```python
from build123d import *

# Parameters (mm, degrees)
SKETCH1_W            = 140
SKETCH1_H            = 92
BOSS_EXTRUDE1_DEPTH  = 6
SKETCH3_R            = 11
SKETCH3_R_2          = 1.6
CUT_EXTRUDE2_DEPTH   = 7
SKETCH6_W            = 10
SKETCH6_H            = 6
CUT_EXTRUDE12_DEPTH  = 4
SKETCH61_W           = 10
SKETCH61_H           = 6
CUT_EXTRUDE14_DEPTH  = 4
SKETCH62_W           = 10
SKETCH62_H           = 6
CUT_EXTRUDE15_DEPTH  = 4
SKETCH63_W           = 10
SKETCH63_H           = 6
CUT_EXTRUDE16_DEPTH  = 4
SKETCH65_W           = 10
SKETCH65_H           = 6
CUT_EXTRUDE17_DEPTH  = 4
SKETCH66_W           = 10
SKETCH66_H           = 6
CUT_EXTRUDE18_DEPTH  = 4
SKETCH67_W           = 10
SKETCH67_H           = 6
CUT_EXTRUDE19_DEPTH  = 4
SKETCH68_W           = 10
SKETCH68_H           = 6
CUT_EXTRUDE110_DEPTH = 4
FILLET1_R            = 5


with BuildPart() as part:
    # Sketch1 → Boss-Extrude1 (new body)
    with BuildSketch(Plane(origin=(0, 0, 0), x_dir=(1, 0, 0), z_dir=(0, 1, 0))):
        Rectangle(SKETCH1_W, SKETCH1_H)
    extrude(amount=BOSS_EXTRUDE1_DEPTH)

    # Sketch3 → Cut-Extrude2 (cut, through all)
    with BuildSketch(Plane(origin=(0, 6, 0), x_dir=(1, 0, 0), z_dir=(0, 1, 0))):
        with Locations((49, 0)):
            Circle(SKETCH3_R)
        with Locations((33.5, -15.5)):
            Circle(SKETCH3_R_2)
        with Locations((33.5, 15.5)):
            Circle(SKETCH3_R_2)
        with Locations((64.5, 15.5)):
            Circle(SKETCH3_R_2)
        with Locations((64.5, -15.5)):
            Circle(SKETCH3_R_2)
    extrude(amount=-CUT_EXTRUDE2_DEPTH, mode=Mode.SUBTRACT)

    # Sketch6 → Cut-Extrude12 (cut, symmetric)
    with BuildSketch(Plane(origin=(49.232221392, 3, -81), x_dir=(1, 0, 0), z_dir=(0, 1, 0))):
        with Locations((0.767778608, -44)):
            Rectangle(SKETCH6_W, SKETCH6_H)
    cut_extrude12 = extrude(amount=CUT_EXTRUDE12_DEPTH, both=True, mode=Mode.SUBTRACT)

    # Sketch61 → Cut-Extrude14 (cut, symmetric)
    with BuildSketch(Plane(origin=(15.898888059, 3, -81), x_dir=(1, 0, 0), z_dir=(0, 1, 0))):
        with Locations((0.767778608, -44)):
            Rectangle(SKETCH61_W, SKETCH61_H)
    cut_extrude14 = extrude(amount=CUT_EXTRUDE14_DEPTH, both=True, mode=Mode.SUBTRACT)

    # Sketch62 → Cut-Extrude15 (cut, symmetric)
    with BuildSketch(Plane(origin=(-17.434445274, 3, -81), x_dir=(1, 0, 0), z_dir=(0, 1, 0))):
        with Locations((0.767778608, -44)):
            Rectangle(SKETCH62_W, SKETCH62_H)
    cut_extrude15 = extrude(amount=CUT_EXTRUDE15_DEPTH, both=True, mode=Mode.SUBTRACT)

    # Sketch63 → Cut-Extrude16 (cut, symmetric)
    with BuildSketch(Plane(origin=(-50.767778608, 3, -81), x_dir=(1, 0, 0), z_dir=(0, 1, 0))):
        with Locations((0.767778608, -44)):
            Rectangle(SKETCH63_W, SKETCH63_H)
    cut_extrude16 = extrude(amount=CUT_EXTRUDE16_DEPTH, both=True, mode=Mode.SUBTRACT)

    # Sketch65 → Cut-Extrude17 (cut, symmetric)
    with BuildSketch(Plane(origin=(49.232221392, 3, -67), x_dir=(1, 0, 0), z_dir=(0, 1, 0))):
        with Locations((0.767778608, -44)):
            Rectangle(SKETCH65_W, SKETCH65_H)
    cut_extrude17 = extrude(amount=CUT_EXTRUDE17_DEPTH, both=True, mode=Mode.SUBTRACT)

    # Sketch66 → Cut-Extrude18 (cut, symmetric)
    with BuildSketch(Plane(origin=(15.898888059, 3, -67), x_dir=(1, 0, 0), z_dir=(0, 1, 0))):
        with Locations((0.767778608, -44)):
            Rectangle(SKETCH66_W, SKETCH66_H)
    cut_extrude18 = extrude(amount=CUT_EXTRUDE18_DEPTH, both=True, mode=Mode.SUBTRACT)

    # Sketch67 → Cut-Extrude19 (cut, symmetric)
    with BuildSketch(Plane(origin=(-17.434445274, 3, -67), x_dir=(1, 0, 0), z_dir=(0, 1, 0))):
        with Locations((0.767778608, -44)):
            Rectangle(SKETCH67_W, SKETCH67_H)
    cut_extrude19 = extrude(amount=CUT_EXTRUDE19_DEPTH, both=True, mode=Mode.SUBTRACT)

    # Sketch68 → Cut-Extrude110 (cut, symmetric)
    with BuildSketch(Plane(origin=(-50.767778608, 3, -67), x_dir=(1, 0, 0), z_dir=(0, 1, 0))):
        with Locations((0.767778608, -44)):
            Rectangle(SKETCH68_W, SKETCH68_H)
    cut_extrude110 = extrude(amount=CUT_EXTRUDE110_DEPTH, both=True, mode=Mode.SUBTRACT)

    # Mirror1: Cut-Extrude12, Cut-Extrude14, Cut-Extrude15, Cut-Extrude16, Cut-Extrude17, Cut-Extrude18, Cut-Extrude19, Cut-Extrude110 across plane
    add(cut_extrude12.mirror(Plane.XY), mode=Mode.SUBTRACT)
    add(cut_extrude14.mirror(Plane.XY), mode=Mode.SUBTRACT)
    add(cut_extrude15.mirror(Plane.XY), mode=Mode.SUBTRACT)
    add(cut_extrude16.mirror(Plane.XY), mode=Mode.SUBTRACT)
    add(cut_extrude17.mirror(Plane.XY), mode=Mode.SUBTRACT)
    add(cut_extrude18.mirror(Plane.XY), mode=Mode.SUBTRACT)
    add(cut_extrude19.mirror(Plane.XY), mode=Mode.SUBTRACT)
    add(cut_extrude110.mirror(Plane.XY), mode=Mode.SUBTRACT)

    # Fillet1
    fillet1_edges = [part.edges().sort_by_distance(p)[0] for p in [
        (70, 3, 46),
        (-70, 3, 46),
        (-70, 3, -46),
        (70, 3, -46),
    ]]
    fillet(fillet1_edges, radius=FILLET1_R)


solid = part.part
```
CAD build for the part. Positions are in the model's coordinates, mm. A direction names the side the tool comes from. Give positions to 0.01 mm unless a question says otherwise; leave off trailing zeros. Loops run counter-clockwise (first coordinate to the right, second up) from the corner with the lowest first, then second, coordinate; pieces in that order, holes last. Notation, with made-up numbers: (15, 55.25) -> (65, 55.25) arc R24 cw to (65, 89.25) -> close; hole circle Ø5 at (23, 5). An arc over 180 degrees is marked (long way). Use a Markdown table: item, result.
1. Slice it at A-A (z = 15.5). List the corners of the cut face in (x, y).
Check result:
| item | result |
|---|---|
| outline | (-70, 0) -> (31.9, 0) -> (31.9, 6) -> (-70, 6) -> close; (35.1, 0) -> (62.9, 0) -> (62.9, 6) -> (35.1, 6) -> close; (66.1, 0) -> (70, 0) -> (70, 6) -> (66.1, 6) -> close |
2. Which spindle directions (+Z, -Z, +X, -X, +Y, -Y) get a long thin tool onto all of the face, cutting with end or side? Do faces 1 (the cylindrical face through (68, 3, 45)), 2 (the flat face through (45, 3, -23)). Say none if no direction does.
Check result:
| item | result |
|---|---|
| face 1 | +Z, +X, +Y, -Y |
| face 2 | +Y, -Y |
3. Slice it at C-C (z = -36.5). List the corners of the cut face in (x, y).
Check result:
| item | result |
|---|---|
| outline | (-70, 0) -> (-55, 0) -> (-55, 6) -> (-70, 6) -> close; (-45, 0) -> (-21.67, 0) -> (-21.67, 6) -> (-45, 6) -> close; (-11.67, 0) -> (11.67, 0) -> (11.67, 6) -> (-11.67, 6) -> close; (21.67, 0) -> (45, 0) -> (45, 6) -> (21.67, 6) -> close; (55, 0) -> (70, 0) -> (70, 6) -> (55, 6) -> close |
4. Slice it at D-D (x = 33.5). List the corners of the cut face in (y, z).
Check result:
| item | result |
|---|---|
| outline | (0, -46) -> (6, -46) -> (6, -17.1) -> (0, -17.1) -> close; (0, -13.9) -> (6, -13.9) -> (6, 13.9) -> (0, 13.9) -> close; (0, 17.1) -> (6, 17.1) -> (6, 46) -> (0, 46) -> close |
5. Slice it at B-B (x = 15.5). List the corners of the cut face in (y, z).
Check result:
| item | result |
|---|---|
| outline | (0, -46) -> (6, -46) -> (6, -40) -> (0, -40) -> close; (0, -34) -> (6, -34) -> (6, -26) -> (0, -26) -> close; (0, -20) -> (6, -20) -> (6, 20) -> (0, 20) -> close; (0, 26) -> (6, 26) -> (6, 34) -> (0, 34) -> close; (0, 40) -> (6, 40) -> (6, 46) -> (0, 46) -> close |
6. Wall check: L1, parallel to Z at x = 49, y = 3.9; L2, parallel to Z at x = 33.5, y = 2; L3, parallel to X at y = 0.5, z = -24.5. Give the ranges that are in metal, low to high. Write a range as [from, to].
Check result:
| item | result |
|---|---|
| L1 | z = [-46, -40], [-34, -26], [-20, -11], [11, 20], [26, 34], [40, 46] |
| L2 | z = [-46, -17.1], [-13.9, 13.9], [17.1, 46] |
| L3 | x = [-70, -55], [-45, -21.67], [-11.67, 11.67], [21.67, 45], [55, 70] |
7. Flat gauge pin, fed straight in: pin 1 (2 mm diameter, centred on x = -6.5, z = -10, fed in from -Y). Where does the tip first touch, or does it go through?
Check result:
| item | result |
|---|---|
| pin 1 | stops at y = 0 |
